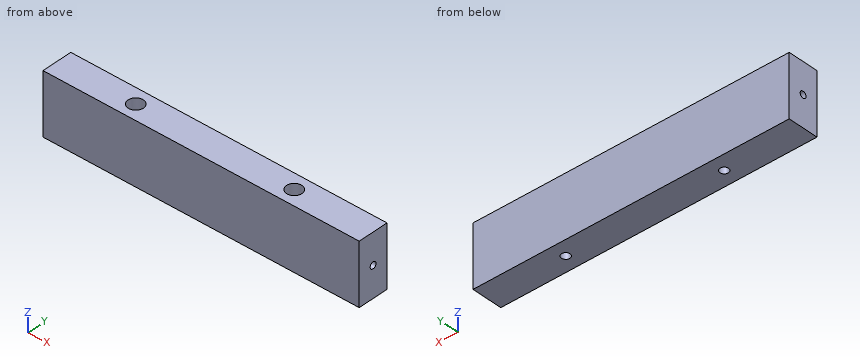
```python
from build123d import *

# Parameters (mm, degrees)
F0_W           = 12.7
F0_H           = 25.4
F1_DEPTH       = 131
F3_D           = 3.5
F3_CBORE_D     = 6.35
F3_CBORE_DEPTH = 18.4
F5_D           = 2.7051
F5_DEPTH       = 12.7
F5_TIP         = 0.8126940303
F7_D           = 2.7051
F7_DEPTH       = 12.7
F7_TIP         = 0.8126940303


with BuildPart() as f1:
    # F0 (on Right) → F1 (new body)
    with BuildSketch(Plane.YZ):
        Rectangle(F0_W, F0_H)
    extrude(amount=F1_DEPTH)

    # F3 (through all)
    with Locations(Plane.XY.offset(12.7)):
        with Locations((32.675, 0), (98.325, 0)):
            CounterBoreHole(F3_D / 2, F3_CBORE_D / 2, F3_CBORE_DEPTH)

    # F5
    with Locations(Plane.YZ.offset(131)):
        with Locations((0, 0)):
            Hole(F5_D / 2, depth=F5_DEPTH)
            with Locations((0, 0, -(F5_DEPTH + F5_TIP / 2))):  # 118° drill point
                Cone(0, F5_D / 2, F5_TIP, mode=Mode.SUBTRACT)

    # F7
    with Locations(Plane(origin=(0, 0, 0), x_dir=(0, -1, 0), z_dir=(-1, 0, 0))):
        with Locations((0, 0)):
            Hole(F7_D / 2, depth=F7_DEPTH)
            with Locations((0, 0, -(F7_DEPTH + F7_TIP / 2))):  # 118° drill point
                Cone(0, F7_D / 2, F7_TIP, mode=Mode.SUBTRACT)


solid = f1.part
```
Read the model definition and answer for the solid it produces. Units are mm, in the model's axes. Give positions to 0.01 mm unless a question says otherwise; leave off trailing zeros. Write each loop counter-clockwise with the first axis right and the second up, starting at its lowest first coordinate (ties: lowest second). Pieces come first, ordered by that corner, then holes. Notation, with made-up numbers: (-24.5, 1.25) -> (-11.5, 1.25) arc R17 cw to (-11.5, 22.25) -> close; hole circle Ø4 at (66.25, 60.5). An arc over 180 degrees is marked (long way). Answer as a JSON object with one key per item and string values.
1) Flat-ended cylindrical pins translate along their axes: pin 1 Ø2.5 at (y, z) = (0, 0) entering from -X; pin 2 Ø5.5 at (x, y) = (98.325, 0) entering from +Z; pin 3 Ø2 at (x, y) = (98.325, 0) entering from -Z. Find the tip coordinate at first contact, or state that the pin passes through.
Findings below:
{"pin 1": "stops at x = 12.76", "pin 2": "stops at z = -5.7", "pin 3": "passes through"}
2) Straight lines are drawn through the part: probe 1 along Z at (x, y) = (8.75, 0); probe 2 along X at (y, z) = (0.75, 7); probe 3 along X at (y, z) = (1.25, 5.5). For each, find the intervals that lie inside material, in ascending order. Write a range as from..to.
Findings below:
{"probe 1": "z = -12.7..-1.35, 1.35..12.7", "probe 2": "x = 0..29.59, 35.76..95.24, 101.41..131", "probe 3": "x = 0..29.76, 35.59..95.41, 101.24..131"}
3) Section A-A on z = 3 is taken. Write down the section's boundary in (x, y) (3 decimals), then the cut area to 3 significant figures.
Findings below:
{"outline": "(0, -6.35) -> (131, -6.35) -> (131, 6.35) -> (0, 6.35) -> close; hole circle Ø6.35 at (32.675, 0); hole circle Ø6.35 at (98.325, 0)", "area": "1,600 mm^2"}
